Design review of the part built by this model. Coordinates are the model's own, in mm. Round coordinates to 2 decimals unless told otherwise and drop trailing zeros. Loops run counter-clockwise (first coordinate to the right, second up) from the corner with the lowest first, then second, coordinate; pieces in that order, holes last. Notation, with made-up numbers: (7.25, 60) - (13.25, 60) arc R11 cw to (13.25, 66) - close; hole circle Ø7 at (44.25, -9.75). An arc over 180 degrees is marked (long way). Return JSON: item names as keys, results as strings. Group by question number.
Autodesk Inventor part; units mm, degrees
ref_plane "YZ Plane" through (0, 0, 0) normal (1, 0, 0) x (0, 1, 0)
ref_plane "XZ Plane" through (0, 0, 0) normal (0, 1, 0) x (-1, 0, 0)
ref_plane "XY Plane" through (0, 0, 0) normal (0, 0, 1) x (1, 0, 0)
sketch "Sketch1" plane through (0, 0, 0) normal (0, 0, 1) x (1, 0, 0)
  line L0 (0, 0) -> (241.3, 0)
  line L1 (241.3, 0) -> (241.3, 101.6)
  line L2 (241.3, 101.6) -> (0, 101.6)
  line L3 (0, 101.6) -> (0, 0)
  circle A0 centre (98.425, 50.8) radius 3.175
  circle A1 centre (142.875, 50.8) radius 3.175
  dimension "d0" = 241.3
  dimension "d1" = 101.6
  dimension "d2" = 6.35
  dimension "d3" = 6.35
  dimension "d4" = 44.45
  dimension "d5" = 98.425
  dimension "d6" = 50.8
extrude "Extrusion1" add sketch "Sketch1" along normal blind 3.175
sketch "Sketch2" plane through (0, 0, 0) normal (-1, 0, 0) x (0, 0, 1)
  line L0 (0, -0.8069) -> (12.7, -0.8069)
  line L1 (12.7, -0.8069) -> (12.7, 151.5931)
  line L2 (12.7, 151.5931) -> (0, 151.5931)
  line L3 (0, 151.5931) -> (0, -0.8069)
  line L4 (0, 101.6) -> (0, 0)
  dimension "d9" = 12.7
  dimension "d10" = 152.4
  dimension "d11" = 0
extrude "Extrusion2" add sketch "Sketch2" along normal blind 12.7
properties part number "Handle"
Q1. For line 1 (Z direction, x = 66.5, y = 33) (3 decimals); line 2 (Y direction, x = 147, z = 2.25); line 3 (X direction, y = 133.5, z = 1.5), list the stretches that pass through material, from the lowest coordinate up.
Q2. Insertion check: pin 1 Ø6.5 at (y, z) = (111.5, 9) entering from +X; pin 2 Ø3.5 at (x, z) = (109, 1) entering from +Y; pin 3 Ø7.5 at (x, y) = (142.875, 50.8) entering from +Z (3 decimals); pin 4 Ø5 at (x, y) = (98.425, 50.8) entering from -Z. Each pin has a flat end and moves straight along its axis. Give the tip position at first contact, or say it passes through.
Q3. Draft analysis for pull direction Y (two halves, no side actions). For faces 1 (the flat face through (-6, -0.807, 6)), 2 (the flat face through (119, 52, 3.175)), 3 (the flat face through (-6, 151.593, 6)), 4 (the cylindrical face through (140.535, 48.654, 1.565)), state which applies: pulls with the +Y half, pulls with the -Y half, needs draft (parallel to the pull), parting line crosses it, or undercut.
Q4. Add section B-B, the plane y = 26.5. State the section outline as (x, z) points (3 decimals), plus the area to 3 significant figures.
Q5. Add section D-D, the plane x = 123. State the section outline as (y, z) points (3 decimals).
Q6. Add section C-C, the plane z = 6. State the section outline as (x, y) points, plus the area to 3 significant figures.
Q7. Add section A-A, the plane y = 50.8. State the section outline as (x, z) points (3 decimals), plus the area to 3 significant figures.
Evaluation:
{
 "1": {"line 1": "0 to 3.175", "line 2": "0 to 101.6", "line 3": "-12.7 to 0"},
 "2": {"pin 1": "x = 0", "pin 2": "y = 101.6", "pin 3": "z = 3.175", "pin 4": "through"},
 "3": {"face 1": "pulls with the -Y half", "face 2": "needs draft", "face 3": "pulls with the +Y half", "face 4": "undercut"},
 "4": {"outline": "(-12.7, 0) - (241.3, 0) - (241.3, 3.175) - (0, 3.175) - (0, 12.7) - (-12.7, 12.7) - close", "area": "927 mm²"},
 "5": {"outline": "(0, 0) - (101.6, 0) - (101.6, 3.175) - (0, 3.175) - close"},
 "6": {"outline": "(-12.7, -0.81) - (0, -0.81) - (0, 151.59) - (-12.7, 151.59) - close", "area": "1,940 mm²"},
 "7": {"outline": "(-12.7, 0) - (95.25, 0) - (95.25, 3.175) - (0, 3.175) - (0, 12.7) - (-12.7, 12.7) - close; (101.6, 0) - (139.7, 0) - (139.7, 3.175) - (101.6, 3.175) - close; (146.05, 0) - (241.3, 0) - (241.3, 3.175) - (146.05, 3.175) - close", "area": "887 mm²"}
}
